Source: CAD feature listing. Evaluate the final solid. Frame: model axes, mm. A direction names the side the tool comes from. Coordinates: 2 decimals unless noted, no trailing zeros. Loops run counter-clockwise (first coordinate to the right, second up) from the corner with the lowest first, then second, coordinate; pieces in that order, holes last. Notation, with made-up numbers: (-16.75, 49.5) - (-12.75, 49.5) arc R24 cw to (-12.75, 66.5) - close; hole circle Ø10 at (-16, -34.5). An arc over 180 degrees is marked (long way). Use CSV: the item, a comma, the result in double quotes. Start each with the question number.
```python
from build123d import *

# Parameters (mm, degrees)
SKETCH_1_W          = 14.9
SKETCH_1_H          = 5.75
EXTRUDE_1_DEPTH     = 7
SKETCH_2_W          = 0.64
SKETCH_2_H          = 0.64
EXTRUDE_2_DEPTH     = 3.4
SKETCH_3_W          = 12.9
SKETCH_3_H          = 3.75
CUT_EXTRUDE_1_DEPTH = 5


with BuildPart() as part:
    # Эскиз1 → Бобышка-Вытянуть1 (new body)
    with BuildSketch(Plane.XY):
        Rectangle(SKETCH_1_W, SKETCH_1_H)
    extrude(amount=EXTRUDE_1_DEPTH)

    # Эскиз2 → Бобышка-Вытянуть2 (add)
    with BuildSketch(Plane.XY.offset(7)):
        with Locations((-2.5, -0.525)):
            Rectangle(SKETCH_2_W, SKETCH_2_H)
        with Locations((-5, -0.525)):
            Rectangle(SKETCH_2_W, SKETCH_2_H)
        with Locations((0, -0.525)):
            Rectangle(SKETCH_2_W, SKETCH_2_H)
        with Locations((2.5, -0.525)):
            Rectangle(SKETCH_2_W, SKETCH_2_H)
        with Locations((5, -0.525)):
            Rectangle(SKETCH_2_W, SKETCH_2_H)
    extrude(amount=EXTRUDE_2_DEPTH)

    # Эскиз3 → Вырез-Вытянуть1 (cut)
    with BuildSketch(Plane(origin=(0, 0, 0), x_dir=(-1, 0, 0), z_dir=(0, 0, -1))):
        Rectangle(SKETCH_3_W, SKETCH_3_H)
    extrude(amount=-CUT_EXTRUDE_1_DEPTH, mode=Mode.SUBTRACT)


solid = part.part
```
(1) Pin query (flat end, axial travel): pin 1 Ø0.7 at (y, z) = (-0.5, 8.5) entering from +X; pin 2 Ø0.7 at (x, z) = (-2.5, 9) entering from +Y (3 decimals); pin 3 Ø1 at (x, y) = (2.5, 1) entering from +Z. Return the tip coordinate at first contact, or that it passes through.
(2) Draft query along X for faces 3 (the flat face through (7.45, 0, 3)), 4 (the flat face through (-6.45, 0, 2)), 5 (the flat face through (-7.45, 0, 3)). Return one class per face: released by +X, released by -X, zero draft, split by the parting line, or undercut.
(3) Section B-B on x = -0.75. Output: boundary loops of the cut face in (y, z) (3 decimals).
(4) Section A-A on z = 8.75. Output: boundary loops of the cut face in (x, y) (3 decimals), plus the area to 3 significant figures.
(5) Section D-D on z = 3. Output: boundary loops of the cut face in (x, y) (3 decimals), plus the area to 3 significant figures.
(6) Section C-C on y = 1.5. Output: boundary loops of the cut face in (x, z).
(7) Ray query, line 1 (Y direction, x = -2, z = 4.25) (3 decimals); line 2 (Z direction, x = 6.25, y = 1.1); line 3 (Z direction, x = -6.5, y = -2.05). Return the intervals inside material, ascending. Write a range as [from, to].
(8) Reachability of faces 1 (the flat face through (0, 1.875, 2)), 2 (the flat face through (0, 2.875, 3)) from +Z, -Z, +X, -X, +Y, -Y: full face, straight path, thin tool, end or side. Return the list, or none.
Solution:
1,pin 1,"stops at x = 5.32"
1,pin 2,"stops at y = -0.205"
1,pin 3,"stops at z = 7"
2,face 3,"released by +X"
2,face 4,"undercut"
2,face 5,"released by -X"
3,outline,"(-2.875, 0) - (-1.875, 0) - (-1.875, 5) - (1.875, 5) - (1.875, 0) - (2.875, 0) - (2.875, 7) - (-2.875, 7) - close"
4,outline,"(-5.32, -0.845) - (-4.68, -0.845) - (-4.68, -0.205) - (-5.32, -0.205) - close; (-2.82, -0.845) - (-2.18, -0.845) - (-2.18, -0.205) - (-2.82, -0.205) - close; (-0.32, -0.845) - (0.32, -0.845) - (0.32, -0.205) - (-0.32, -0.205) - close; (2.18, -0.845) - (2.82, -0.845) - (2.82, -0.205) - (2.18, -0.205) - close; (4.68, -0.845) - (5.32, -0.845) - (5.32, -0.205) - (4.68, -0.205) - close"
4,area,"2.05 mm²"
5,outline,"(-7.45, -2.875) - (7.45, -2.875) - (7.45, 2.875) - (-7.45, 2.875) - close; hole (-6.45, -1.875) - (6.45, -1.875) - (6.45, 1.875) - (-6.45, 1.875) - close"
5,area,"37.3 mm²"
6,outline,"(-7.45, 0) - (-6.45, 0) - (-6.45, 5) - (6.45, 5) - (6.45, 0) - (7.45, 0) - (7.45, 7) - (-7.45, 7) - close"
7,line 1,"y = [-2.875, -1.875], [1.875, 2.875]"
7,line 2,"z = [5, 7]"
7,line 3,"z = [0, 7]"
8,face 1,"-Z"
8,face 2,"+Z, -Z, +X, -X, +Y"
